Verification items for the finished model (mm, model axes). A direction names the side the tool comes from. Round coordinates to 2 decimals unless told otherwise and drop trailing zeros. Order: outer loops, then holes, each group sorted by start corner. A loop starts at its lowest first (then second) coordinate and runs counter-clockwise, first axis right, second up. Notation, with made-up numbers: (-31.5, 15) -> (18.5, 15) arc R26 ccw to (18.5, 41) -> close; hole circle Ø6 at (44.25, 28.5). An arc over 180 degrees is marked (long way). Return JSON: item names as keys, results as strings. Group by question number.
1) Section check A-A on y = 32. Enter the section's corners in (x, z).
2) Scan lines: L1, parallel to X at y = 25.9, z = 0; L2, parallel to X at y = 25.5, z = -3; L3, parallel to X at y = 4.15, z = 0. Record each from-to range of solid material in increasing order.
3) Section check B-B on y = 17. Enter the section's corners in (x, z).
4) Tool access check on faces 1 (the cylindrical face through (-1.802, 32.056, -5.723)), 2 (the flat face through (8, 31, 0)), 3 (the cylindrical face through (-2.23, 3.29, 2.43)). Record the directions out of +Z, -Z, +X, -X, +Y, -Y that give a thin tool (end or side, any length) a straight path to the whole face; none if there is none.
5) Depth check by flat-ended pin: pin 1 (5.5 mm diameter, centred on x = -1, z = 2, fed in from -Y); pin 2 (6 mm diameter, centred on y = 13, z = -6.5, fed in from +X); pin 3 (1 mm diameter, centred on x = 1.5, y = 23.5, fed in from +Z); pin 4 (1.5 mm diameter, centred on y = 19, z = -4, fed in from +X). Enter the tip coordinate at first touch or a pass-through.
6) Draft check along Z on faces 4 (the flat face through (-8, 31, 0)), 5 (the flat face through (4, 28, 0)), 6 (the cylindrical face through (0, 31, 9)). Enter one of: pulls with the +Z half, pulls with the -Z half, needs draft (parallel to the pull), parting line crosses it, or undercut.
```python
from build123d import *

# Parameters (mm, degrees)
ENL_V_MAT_EXTRU_1_DEPTH = 40.127995093
CHANFREIN1_SIZE         = 1
CHANFREIN2_SIZE         = 0.5
CHANFREIN3_SIZE         = 1


with BuildPart() as part:
    # Esquisse1 → Révolution1 (revolve)
    with BuildSketch(Plane.XY, mode=Mode.PRIVATE) as r_volution1_sk:
        Polygon((3.3, 6), (2.5, 6), (2.5, 22), (3.3, 22), (3.3, 28), (6, 28), (6, 37), (9, 37), (9, 25), (7.56, 25), (7.56, 26.25), (5.41, 26.25), (5.41, 25), (5, 25), (5, 0), (3.3, 0), align=None)
    revolve(r_volution1_sk.sketch.rotate(Axis((0, 0, 0), (0, 1, 0)), 90), axis=Axis((0, 0, 0), (0, 1, 0)))

    # Esquisse2 → Enlèv. mat.-Extru.1 (cut, through all)
    with BuildSketch(Plane(origin=(0, 37, 0), x_dir=(1, 0, 0), z_dir=(0, 1, 0))):
        with BuildLine():
            Line((-8, 4.123105626), (-8, -4.123105626))
            ThreePointArc((-8, -4.123105626), (-9, 0), (-8, 4.123105626))
        make_face()
        with BuildLine():
            Line((8, 4.123105626), (8, -4.123105626))
            ThreePointArc((8, -4.123105626), (9, 0), (8, 4.123105626))
        make_face()
    extrude(amount=-ENL_V_MAT_EXTRU_1_DEPTH, mode=Mode.SUBTRACT)

    # Chanfrein1
    chanfrein1_edges = [part.edges().sort_by_distance(p)[0] for p in [
        (0, 37, 6),
    ]]
    chamfer(chanfrein1_edges, length=CHANFREIN1_SIZE)

    # Chanfrein2
    chanfrein2_edges = [part.edges().sort_by_distance(p)[0] for p in [
        (0, 6, 2.5),
        (0, 22, 2.5),
        (0, 28, 3.3),
        (0, 0, 3.3),
    ]]
    chamfer(chanfrein2_edges, length=CHANFREIN2_SIZE)

    # Chanfrein3
    chanfrein3_edges = [part.edges().sort_by_distance(p)[0] for p in [
        (0, 0, 5),
    ]]
    chamfer(chanfrein3_edges, length=CHANFREIN3_SIZE)


solid = part.part
```
Check result:
{
 "1": {"outline": "(-8, -4.12) arc R9 ccw to (8, -4.12) -> (8, 4.12) arc R9 ccw to (-8, 4.12) -> close; hole circle Ø12 at (0, 0)"},
 "2": {"L1": "-8 to -7.56, -5.41 to -3.3, 3.3 to 5.41, 7.56 to 8", "L2": "-8 to -6.94, -4.5 to -1.37, 1.37 to 4.5, 6.94 to 8", "L3": "-5 to -3.3, 3.3 to 5"},
 "3": {"outline": "circle Ø10 at (0, 0); hole circle Ø5 at (0, 0)"},
 "4": {"face 1": "+Y", "face 2": "+Z, -Z, +X, +Y, -Y", "face 3": "-Y"},
 "5": {"pin 1": "y = 0", "pin 2": "x = 3.57", "pin 3": "z = 4.9", "pin 4": "x = 3.8"},
 "6": {"face 4": "needs draft", "face 5": "undercut", "face 6": "pulls with the +Z half"}
}
